```python
from build123d import *

# Parameters (mm, degrees)
F0_W      = 30
F0_H      = 30
F1_DEPTH  = 10
F2_R      = 9.55
F3_DEPTH  = 7
F4_R      = 6.75
F5_DEPTH  = 3
F7_DEPTH  = 10
F8_R      = 1.5
F9_DEPTH  = 8
F10_R     = 1.5
F11_DEPTH = 8
F12_R     = 1
F13_DEPTH = 10


with BuildPart() as f1:
    # F0 (on Top) → F1 (new body)
    with BuildSketch(Plane.XY):
        with Locations((15, -15)):
            Rectangle(F0_W, F0_H)
    extrude(amount=-F1_DEPTH)

    # F2 (on face) → F3 (cut)
    with BuildSketch(Plane.XY):
        with Locations((15, -15)):
            Circle(F2_R)
    extrude(amount=-F3_DEPTH, mode=Mode.SUBTRACT)

    # F4 (on face) → F5 (cut, through all)
    with BuildSketch(Plane.XY.offset(-7)):
        with Locations((15, -15)):
            Circle(F4_R)
    extrude(amount=-F5_DEPTH, mode=Mode.SUBTRACT)

    # F6 (on face) → F7 (cut, through all)
    with BuildSketch(Plane.XY):
        with BuildLine():
            ThreePointArc((1.95, -15), (3.5, -16.55), (5.05, -15))
            ThreePointArc((5.05, -15), (3.5, -13.45), (1.95, -15))
        make_face()
    extrude(amount=-F7_DEPTH, mode=Mode.SUBTRACT)

    # F8 (on face) → F9 (cut)
    with BuildSketch(Plane.XZ.offset(30)):
        with Locations((5, -5)):
            Circle(F8_R)
        with Locations((25, -5)):
            Circle(F8_R)
    extrude(amount=-F9_DEPTH, mode=Mode.SUBTRACT)

    # F10 (on face) → F11 (cut)
    with BuildSketch(Plane(origin=(0, 0, 0), x_dir=(-1, 0, 0), z_dir=(0, 1, 0))):
        with Locations((-25, -5)):
            Circle(F10_R)
        with Locations((-5, -5)):
            Circle(F10_R)
    extrude(amount=-F11_DEPTH, mode=Mode.SUBTRACT)

    # F12 (on face) → F13 (cut, through all)
    with BuildSketch(Plane(origin=(0, 0, -10), x_dir=(1, 0, 0), z_dir=(0, 0, -1))):
        with Locations((9, 4)):
            Circle(F12_R)
        with Locations((21, 4)):
            Circle(F12_R)
        with Locations((21, 26)):
            Circle(F12_R)
        with Locations((9, 26)):
            Circle(F12_R)
    extrude(amount=-F13_DEPTH, mode=Mode.SUBTRACT)


solid = f1.part
```
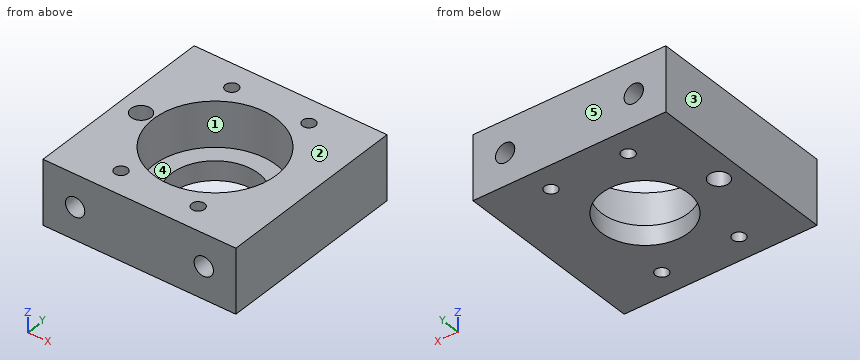
For this review, take the finished solid that the model builds, in its own axes (mm). Face numbers are marked on the shaded views. A direction names the side the tool comes from. Give positions to 0.01 mm unless a question says otherwise; leave off trailing zeros. Write each loop counter-clockwise with the first axis right and the second up, starting at its lowest first coordinate (ties: lowest second). Pieces come first, ordered by that corner, then holes.
Item 1: Take a section at B-B (x = 15). Give the boundary of the cut face in (y, z).
Item 2: Take a section at D-D (z = -1.5). Give the boundary of the cut face in (x, y), and give its area (3 significant figures).
Item 3: The part is to be moulded in two halves that separate along Y. For the marked faces 3, 4 and 5, say which applies: +Y half, -Y half, draft (parallel to the pull), parting line (faces both ways), or undercut.
Item 4: Take a section at A-A (y = -26). Give the boundary of the cut face in (x, z).
Item 5: Wall thickness on probe 1 along X at (y, z) = (-4, -2.75); probe 2 along Y at (x, z) = (15, -7.75); probe 3 along Z at (x, y) = (25, -26.75): over which ranges is each line inside the solid? List them lowest first.
Item 6: Insertion check: P1, Ø1.5, axis at x = 5, z = -5.5, coming from the -Y side; P2, Ø1.5, axis at x = 5, z = -5.5, coming from the +Y side. Each pin has a flat end and moves straight along its axis. Give the tip position at first contact, or say it passes through.
Item 7: Machinability: for the marked faces 1 and 2, which of the approach directions +Z, -Z, +X, -X, +Y, -Y give a long, thin tool a straight path to every point of the face, cutting with its end or side? Answer none if there is none.
Item 8: Take a section at C-C (y = -15). Give the boundary of the cut face in (x, z).
Established:
1. outline: (-30, -10) - (-21.75, -10) - (-21.75, -7) - (-24.55, -7) - (-24.55, 0) - (-30, 0) - close; (-8.25, -10) - (0, -10) - (0, 0) - (-5.45, 0) - (-5.45, -7) - (-8.25, -7) - close
2. outline: (0, -30) - (30, -30) - (30, 0) - (0, 0) - close; hole circle Ø3.1 at (3.5, -15); hole circle Ø19.1 at (15, -15); hole circle Ø2 at (9, -26); hole circle Ø2 at (9, -4); hole circle Ø2 at (21, -26); hole circle Ø2 at (21, -4)
2. area: 593 mm2
3. face 3: draft
3. face 4: undercut
3. face 5: +Y half
4. outline: (0, -10) - (8, -10) - (8, 0) - (0, 0) - close; (10, -10) - (20, -10) - (20, 0) - (10, 0) - close; (22, -10) - (30, -10) - (30, 0) - (22, 0) - close; hole circle Ø3 at (5, -5); hole circle Ø3 at (25, -5)
5. probe 1: x = 0 to 8, 10 to 20, 22 to 30
5. probe 2: y = -30 to -21.75, -8.25 to 0
5. probe 3: z = -10 to -6.5, -3.5 to 0
6. P1: stops at y = -22
6. P2: stops at y = -8
7. face 1: +Z
7. face 2: +Z, +X, -X, +Y, -Y
8. outline: (0, -10) - (1.95, -10) - (1.95, 0) - (0, 0) - close; (5.05, -10) - (8.25, -10) - (8.25, -7) - (5.45, -7) - (5.45, 0) - (5.05, 0) - close; (21.75, -10) - (30, -10) - (30, 0) - (24.55, 0) - (24.55, -7) - (21.75, -7) - close
